```python
from build123d import *

# Parameters (mm, degrees)
CROQUIS1_W              = 73
CROQUIS1_H              = 30
SALIENTE_EXTRUIR1_DEPTH = 2
CROQUIS2_R              = 9.975
CROQUIS2_R_2            = 9.95
CROQUIS2_R_3            = 9.75
SALIENTE_EXTRUIR2_DEPTH = 2


with BuildPart() as part:
    # Croquis1 → Saliente-Extruir1 (new body)
    with BuildSketch(Plane(origin=(0, 0, 0), x_dir=(1, 0, 0), z_dir=(0, 1, 0))):
        Rectangle(CROQUIS1_W, CROQUIS1_H)
    extrude(amount=SALIENTE_EXTRUIR1_DEPTH)

    # Croquis2 → Saliente-Extruir2 (add)
    with BuildSketch(Plane(origin=(0, 2, 0), x_dir=(1, 0, 0), z_dir=(0, 1, 0))):
        with Locations(Location((-25, 0, 0), (0, 0, 90))):
            Circle(CROQUIS2_R)
        with Locations(Location((0, 0, 0), (0, 0, 90))):
            Circle(CROQUIS2_R_2)
        with Locations(Location((25, 0, 0), (0, 0, 90))):
            Circle(CROQUIS2_R_3)
    extrude(amount=SALIENTE_EXTRUIR2_DEPTH)


solid = part.part
```
Model file for the job. Use its own axes, mm. A direction names the side the tool comes from. Give positions to 0.01 mm unless a question says otherwise; leave off trailing zeros. Write each loop counter-clockwise with the first axis right and the second up, starting at its lowest first coordinate (ties: lowest second). Pieces come first, ordered by that corner, then holes. Notation, with made-up numbers: M 87,67.5 L 131,67.5 A16 ccw 131,95.5 Z; hole C -29,88 d4. An arc over 180 degrees is marked long. Use a Markdown table: item, result.
1) Pull direction X, two halves, no side cores. Call faces 1 (the flat face through (-36.5, 1, 0)), 2 (the cylindrical face through (9.713, 2.986, 2.157)), 3 (the flat face through (-1, 1, -15)), 4 (the flat face through (36.5, 1, 0)): +X half, -X half, draft (parallel to the pull), parting line (faces both ways), or undercut.
Responses:
| item | result |
|---|---|
| face 1 | -X half |
| face 2 | undercut |
| face 3 | draft |
| face 4 | +X half |
2) Cut at C-C (x = 0). List the corners of the cut face in (y, z), and give its area (3 significant figures).
Responses:
| item | result |
|---|---|
| outline | M 0,-15 L 2,-15 L 2,-9.95 L 4,-9.95 L 4,9.95 L 2,9.95 L 2,15 L 0,15 Z |
| area | 99.8 mm2 |
3) Cut at D-D (z = 3.5). List the corners of the cut face in (x, y).
Responses:
| item | result |
|---|---|
| outline | M -36.5,0 L 36.5,0 L 36.5,2 L 34.1,2 L 34.1,4 L 15.9,4 L 15.9,2 L 9.31,2 L 9.31,4 L -9.31,4 L -9.31,2 L -15.66,2 L -15.66,4 L -34.34,4 L -34.34,2 L -36.5,2 Z |
4) Cut at B-B (z = 0). List the corners of the cut face in (x, y) (3 decimals), and give its area (3 significant figures).
Responses:
| item | result |
|---|---|
| outline | M -36.5,0 L 36.5,0 L 36.5,2 L 34.75,2 L 34.75,4 L 15.25,4 L 15.25,2 L 9.95,2 L 9.95,4 L -9.95,4 L -9.95,2 L -15.025,2 L -15.025,4 L -34.975,4 L -34.975,2 L -36.5,2 Z |
| area | 265 mm2 |
5) Pin check, flat tip, straight feed: pin 1 (4 mm diameter, centred on x = -20, z = 11.5, fed in from +Y). Stop position of the tip, or through.
Responses:
| item | result |
|---|---|
| pin 1 | stops at y = 2 |
6) Cut at A-A (x = -25). List the corners of the cut face in (y, z) (3 decimals), and give its area (3 significant figures).
Responses:
| item | result |
|---|---|
| outline | M 0,-15 L 2,-15 L 2,-9.975 L 4,-9.975 L 4,9.975 L 2,9.975 L 2,15 L 0,15 Z |
| area | 99.9 mm2 |
7) Tool access for faces 5 (the flat face through (0, 4, 0)), 6 (the cylindrical face through (34.52, 2.99, 2.11)): list every direction of +Z, -Z, +X, -X, +Y, -Y with a clear straight run to the whole face (end or side of a thin tool).
Responses:
| item | result |
|---|---|
| face 5 | +Z, -Z, +X, -X, +Y |
| face 6 | +Y |
8) Drill centre lines: line 1 (X direction, y = 3.1, z = -2.75); line 2 (X direction, y = 3.7, z = 8.5); line 3 (Y direction, x = 24.5, z = 10.5). Where is each one in solid material? Low to high. Write a range as from..to.
Responses:
| item | result |
|---|---|
| line 1 | x = -34.59..-15.41, -9.56..9.56, 15.65..34.35 |
| line 2 | x = -30.22..-19.78, -5.17..5.17, 20.22..29.78 |
| line 3 | y = 0..2 |
